```python
from build123d import *

# Parameters (mm, degrees)
SKETCH1_W           = 105.87
SKETCH1_H           = 82.04
SKETCH1_W_2         = 88.3
SKETCH1_H_2         = 42.78
BOSS_EXTRUDE1_DEPTH = 4
SKETCH1_4_W         = 97.87
SKETCH1_4_H         = 60.01
SKETCH1_4_W_2       = 88.3
SKETCH1_4_H_2       = 42.78
BOSS_EXTRUDE2_DEPTH = 6.35
SKETCH2_R           = 1.449406475
CUT_EXTRUDE1_DEPTH  = 85.876744687
BOSS_EXTRUDE3_DEPTH = 105.87
FILLET6_R           = 1
BOSS_EXTRUDE4_DEPTH = 2
FILLET7_R           = 1
SKETCH5_W           = 1.65
SKETCH5_H           = 33.3
CUT_EXTRUDE3_DEPTH  = 6.08
BOSS_EXTRUDE6_START = 1.5
SKETCH10_W          = 105.87
SKETCH10_H          = 92.304593272
SKETCH10_R          = 1.449406475
SKETCH10_W_2        = 88.3
SKETCH10_H_2        = 42.78
BOSS_EXTRUDE6_DEPTH = 1.5
BOSS_EXTRUDE7_DEPTH = 105.87
FILLET9_R           = 1
FILLET10_R          = 5


with BuildPart() as part:
    # Sketch1 → Boss-Extrude1 (new body)
    with BuildSketch(Plane(origin=(0, 0, 0), x_dir=(1, 0, 0), z_dir=(0, 1, 0))):
        with Locations((15.929638567, -8.187731543)):
            Rectangle(SKETCH1_W, SKETCH1_H)
        with Locations((15.929638567, -14.302731543)):
            Rectangle(SKETCH1_W_2, SKETCH1_H_2, mode=Mode.SUBTRACT)
    extrude(amount=BOSS_EXTRUDE1_DEPTH)

    # Sketch1<4> → Boss-Extrude2 (add)
    with BuildSketch(Plane(origin=(0, 0, 0), x_dir=(1, 0, 0), z_dir=(0, 1, 0))):
        with Locations((15.929638567, -14.302731543)):
            Rectangle(SKETCH1_4_W, SKETCH1_4_H)
        with Locations((15.929638567, -14.302731543)):
            Rectangle(SKETCH1_4_W_2, SKETCH1_4_H_2, mode=Mode.SUBTRACT)
    extrude(amount=BOSS_EXTRUDE2_DEPTH)

    # Sketch2 → Cut-Extrude1 (cut, through all)
    with BuildSketch(Plane.XZ):
        with Locations(Location((9.192630415, -21.45022355, 0), (0, 0, 270))):
            Circle(SKETCH2_R)
    extrude(amount=-CUT_EXTRUDE1_DEPTH, mode=Mode.SUBTRACT)

    # Sketch3 → Boss-Extrude3 (add)
    with BuildSketch(Plane.ZY.offset(37.005361433)):
        Polygon((-32.832268457, 0), (-49.732268457, 0), (-46.932268457, 4), (-32.832268457, 4), align=None)
    extrude(amount=-BOSS_EXTRUDE3_DEPTH)

    # Fillet6
    fillet6_edges = [part.edges().sort_by_distance(p)[0] for p in [
        (-33.005361433, 6.35, 14.302731543),
        (15.929638567, 6.35, 44.307731543),
        (64.864638567, 6.35, 14.302731543),
        (15.929638567, 6.35, -15.702268457),
    ]]
    fillet(fillet6_edges, radius=FILLET6_R)

    # Sketch4 → Boss-Extrude4 (add)
    with BuildSketch(Plane(origin=(0, 4, 0), x_dir=(1, 0, 0), z_dir=(0, 1, 0))):
        with BuildLine():
            Line((64.864638567, 25.152939827), (-33.005361433, 25.152939827))
            ThreePointArc((-33.005361433, 25.152939827), (-34.005361433, 26.152939827), (-33.005361433, 27.152939827))
            Line((-33.005361433, 27.152939827), (64.864638567, 27.152939827))
            ThreePointArc((64.864638567, 27.152939827), (65.864638567, 26.152939827), (64.864638567, 25.152939827))
        make_face()
        with BuildLine():
            Line((-33.005361433, 41.932268457), (64.864638567, 41.932268457))
            ThreePointArc((64.864638567, 41.932268457), (65.864638567, 42.932268457), (64.864638567, 43.932268457))
            Line((64.864638567, 43.932268457), (-33.005361433, 43.932268457))
            ThreePointArc((-33.005361433, 43.932268457), (-34.005361433, 42.932268457), (-33.005361433, 41.932268457))
        make_face()
        with BuildLine():
            Line((64.864638567, -48.207731543), (-33.005361433, -48.207731543))
            ThreePointArc((-33.005361433, -48.207731543), (-34.005361433, -47.207731543), (-33.005361433, -46.207731543))
            Line((-33.005361433, -46.207731543), (64.864638567, -46.207731543))
            ThreePointArc((64.864638567, -46.207731543), (65.864638567, -47.207731543), (64.864638567, -48.207731543))
        make_face()
    extrude(amount=BOSS_EXTRUDE4_DEPTH)

    # Fillet7
    fillet7_edges = [part.edges().sort_by_distance(p)[0] for p in [
        (65.864638567, 6, 47.207731543),
        (15.929638567, 6, 46.207731543),
        (-34.005361433, 6, 47.207731543),
        (15.929638567, 6, 48.207731543),
        (-34.005361433, 6, -42.932268457),
        (15.929638567, 6, -41.932268457),
        (65.864638567, 6, -42.932268457),
        (15.929638567, 6, -43.932268457),
        (65.864638567, 6, -26.152939827),
        (15.929638567, 6, -27.152939827),
        (-34.005361433, 6, -26.152939827),
        (15.929638567, 6, -25.152939827),
    ]]
    fillet(fillet7_edges, radius=FILLET7_R - 0.0001)  # a hair under: the kernel refuses the full size

    # Sketch5 → Cut-Extrude3 (cut)
    with BuildSketch(Plane(origin=(0, 6.35, 0), x_dir=(1, 0, 0), z_dir=(0, 1, 0))):
        with Locations((-29.045361433, -14.302731543)):
            Rectangle(SKETCH5_W, SKETCH5_H)
    extrude(amount=-CUT_EXTRUDE3_DEPTH, mode=Mode.SUBTRACT)

    # Sketch10 → Boss-Extrude6 (add)
    with BuildSketch(Plane.XZ.offset(BOSS_EXTRUDE6_START)):
        with Locations((15.929638567, 3.055434907)):
            Rectangle(SKETCH10_W, SKETCH10_H)
        with Locations(Location((9.192630415, -21.45022355, 0), (0, 0, 270))):
            Circle(SKETCH10_R, mode=Mode.SUBTRACT)
        with Locations((15.929638567, 14.302731543)):
            Rectangle(SKETCH10_W_2, SKETCH10_H_2, mode=Mode.SUBTRACT)
    extrude(amount=-BOSS_EXTRUDE6_DEPTH)

    # Sketch11 → Boss-Extrude7 (add)
    with BuildSketch(Plane.ZY.offset(37.005361433)):
        Polygon((-49.732268457, 0), (-50.782268457, -1.5), (-43.096861729, -1.5), (-43.096861729, 0), align=None)
    extrude(amount=-BOSS_EXTRUDE7_DEPTH)

    # Fillet9
    fillet9_edges = [part.edges().sort_by_distance(p)[0] for p in [
        (9.192630415, -1.5, -20.000817075),
    ]]
    fillet(fillet9_edges, radius=FILLET9_R)

    # Fillet10
    fillet10_edges = [part.edges().sort_by_distance(p)[0] for p in [
        (-37.005361433, -1.5, -0.787268457),
        (68.864638567, -1.5, -0.787268457),
        (15.929638567, -1.5, 49.207731543),
    ]]
    fillet(fillet10_edges, radius=FILLET10_R)


solid = part.part
```
For this review, take the finished solid that the model builds, in its own axes (mm). A direction names the side the tool comes from. Give positions to 0.01 mm unless a question says otherwise; leave off trailing zeros. Write each loop counter-clockwise with the first axis right and the second up, starting at its lowest first coordinate (ties: lowest second). Pieces come first, ordered by that corner, then holes.
Item 1: The part is to be moulded in two halves that separate along X. For faces 4 (the face through (15, -1.5, -15)), 5 (the face through (-28.22, 0, 14)), 6 (the face through (9.63, 1.72, -22.83)), 7 (the face through (-35.502, -0.074, -1.487)), say which applies: +X half, -X half, draft (parallel to the pull), parting line (faces both ways), or undercut.
Item 2: Take a section at B-B (z = 14.5). Give the boundary of the cut face in (x, y).
Item 3: Insertion check: P1, Ø1.3, axis at x = -29.5, y = 2.5, coming from the +Z side; P2, Ø0.8, axis at x = -29, y = 5, coming from the -Z side; P3, Ø1.1, axis at x = 13.5, y = 4.5, coming from the -Z side. Each pin has a flat end and moves straight along its axis. Give the tip position at first contact, or say it passes through.
Item 4: Take a section at D-D (z = 42). Give the boundary of the cut face in (x, y).
Item 5: Wall thickness on probe 1 along Z at (x, y) = (-21, 4.25); probe 2 along X at (y, z) = (3.5, -7); probe 3 along Z at (x, y) = (-16, 5.25): over which ranges is each line inside the solid? List them lowest first.
Item 6: Machinability: for faces 1 (the face through (15.19, 1.29, -48.83)), 2 (the face through (-29.87, 3, 15)), 3 (the face through (60.08, 2, 14)), which of the approach directions +Z, -Z, +X, -X, +Y, -Y give a long, thin tool a straight path to every point of the face, cutting with its end or side? Answer none if there is none.
Item 7: Take a section at C-C (y = 2.25). Give the boundary of the cut face in (x, z), and give its area (3 significant figures).
Established:
1. face 4: draft
1. face 5: undercut
1. face 6: undercut
1. face 7: -X half
2. outline: (-37.01, 3.5) arc R5 ccw to (-32.01, -1.5) - (-28.22, -1.5) - (-28.22, 0.27) - (-29.87, 0.27) - (-29.87, 6.35) - (-32.01, 6.35) arc R1 ccw to (-33.01, 5.35) - (-33.01, 4) - (-37.01, 4) - close; (60.08, -1.5) - (63.86, -1.5) arc R5 ccw to (68.86, 3.5) - (68.86, 4) - (64.86, 4) - (64.86, 5.35) arc R1 ccw to (63.86, 6.35) - (60.08, 6.35) - close
3. P1: stops at z = 49.2
3. P2: stops at z = -43.93
3. P3: stops at z = -46.97
4. outline: (-37.01, 3.5) arc R5 ccw to (-32.01, -1.5) - (63.86, -1.5) arc R5 ccw to (68.86, 3.5) - (68.86, 4) - (64.86, 4) - (64.86, 5.35) arc R1 ccw to (63.86, 6.35) - (-32.01, 6.35) arc R1 ccw to (-33.01, 5.35) - (-33.01, 4) - (-37.01, 4) - close
5. probe 1: z = -43.93 to -41.93, -27.15 to -25.15, -15.7 to -7.09, 35.69 to 44.31, 46.21 to 48.21
5. probe 2: x = -37.01 to -28.22, 60.08 to 68.86
5. probe 3: z = -43.9 to -41.96, -27.12 to -25.18, -15.7 to -7.09, 35.69 to 44.31, 46.24 to 48.18
6. face 1: -Z, +X, -X, +Y
6. face 2: +Y
6. face 3: +Y, -Y
7. outline: (-36.85, -48.16) - (68.71, -48.16) - (68.71, 49.05) - (-36.85, 49.05) - close; hole (-29.87, -2.35) - (-28.22, -2.35) - (-28.22, -7.09) - (60.08, -7.09) - (60.08, 35.69) - (-28.22, 35.69) - (-28.22, 30.95) - (-29.87, 30.95) - close; hole circle Ø2.9 at (9.19, -21.45)
7. area: 6,420 mm2
